Source: CAD feature listing. Evaluate the final solid. Frame: model axes, mm. A direction names the side the tool comes from. Coordinates: 2 decimals unless noted, no trailing zeros. Write each loop counter-clockwise with the first axis right and the second up, starting at its lowest first coordinate (ties: lowest second). Pieces come first, ordered by that corner, then holes. Notation, with made-up numbers: (-13, 11) - (16, 11) arc R13 cw to (16, 20) - close; hole circle Ø8 at (28.5, -38). An arc over 180 degrees is marked (long way). One line per question, with ' | ' between items. Start each with the question number.
Q1. Cut plane B-B, the plane x = -178.5. Return loops of the section in (y, z), plus the area to 3 significant figures.
Q2. Access query for faces 1 (the face through (-4, 1.143, -1)), 2 (the face through (4, -1.143, -1)). Directions: +Z, -Z, +X, -X, +Y, -Y. A direction counts if a zero-diameter tool reaches every point of the face in a straight line with its end or side. Return the directions, or none.
Q3. Cut plane D-D, the plane x = 21. Return loops of the section in (y, z), plus the area to 3 significant figures.
Q4. Cut plane A-A, the plane z = -6.5. Return loops of the section in (x, y).
Q5. Cut plane C-C, the plane z = 51.5. Return loops of the section in (x, y).
Q6. Line query: line 1 (X direction, y = -0.85, z = -31); line 2 (Y direction, x = 54.5, z = -42); line 3 (X direction, y = 0.2, z = 36). Output: solid intervals per line, ascending.
Q7. Contact query for flat-ended pins moving along their axis: P1, Ø0.8, axis at y = 0, z = -75, coming from the +X side; P2, Ø1.1, axis at x = -317, y = 0.5, coming from the +Z side; P3, Ø0.7, axis at x = 18.5, y = 0, coming from the -Z side. Output: stop coordinate, or through.
```python
from build123d import *

# Parameters (mm, degrees)
SKETCH1_W           = 635.3556
SKETCH1_H           = 145.542
BOSS_EXTRUDE1_DEPTH = 1.143
SKETCH2_W           = 254
SKETCH2_H           = 2.7305
BOSS_EXTRUDE2_DEPTH = 3.175
SKETCH3_W           = 3.175
SKETCH3_H           = 38.1
CUT_EXTRUDE1_DEPTH  = 3.7305
SKETCH4_W           = 2.3368
SKETCH4_H           = 72.771
CUT_EXTRUDE2_DEPTH  = 3.7305


with BuildPart() as part:
    # Sketch1 → Boss-Extrude1 (new body, symmetric)
    with BuildSketch(Plane(origin=(0, 0, 0), x_dir=(1, 0, 0), z_dir=(0, 1, 0))):
        Rectangle(SKETCH1_W, SKETCH1_H)
    extrude(amount=BOSS_EXTRUDE1_DEPTH, both=True)

    # Sketch2 → Boss-Extrude2 (add)
    with BuildSketch(Plane(origin=(0, 0, -72.771), x_dir=(-1, 0, 0), z_dir=(0, 0, -1))):
        with Locations((-157.8229, 0.22225)):
            Rectangle(SKETCH2_W, SKETCH2_H)
        with Locations((157.8229, 0.22225)):
            Rectangle(SKETCH2_W, SKETCH2_H)
    extrude(amount=BOSS_EXTRUDE2_DEPTH)

    # Sketch3 → Cut-Extrude1 (cut, through all)
    with BuildSketch(Plane.XZ.offset(1.143)):
        with Locations((-316.0903, 53.721)):
            Rectangle(SKETCH3_W, SKETCH3_H)
    cut_extrude1 = extrude(amount=-CUT_EXTRUDE1_DEPTH, mode=Mode.SUBTRACT)

    # Mirror1: Cut-Extrude1 across plane
    add(cut_extrude1.mirror(Plane(origin=(0, 0, 0), x_dir=(0, 0, 1), z_dir=(1, 0, 0))), mode=Mode.SUBTRACT)

    # Sketch4 → Cut-Extrude2 (cut, through all)
    with BuildSketch(Plane.XZ.offset(1.143)):
        with Locations((0.0254, -36.3855)):
            Rectangle(SKETCH4_W, SKETCH4_H)
    extrude(amount=-CUT_EXTRUDE2_DEPTH, mode=Mode.SUBTRACT)


solid = part.part
```
Reply:
1) outline: (-1.14, -75.95) - (1.59, -75.95) - (1.59, -72.77) - (1.14, -72.77) - (1.14, 72.77) - (-1.14, 72.77) - close | area: 341 mm^2
2) face 1: +Z, +X, -X, +Y | face 2: +Z, -Z, +X, -X, -Y
3) outline: (-1.14, -72.77) - (1.14, -72.77) - (1.14, 72.77) - (-1.14, 72.77) - close | area: 333 mm^2
4) outline: (-317.68, -1.14) - (-1.14, -1.14) - (-1.14, 1.14) - (-317.68, 1.14) - close; (1.19, -1.14) - (317.68, -1.14) - (317.68, 1.14) - (1.19, 1.14) - close
5) outline: (-314.5, -1.14) - (314.5, -1.14) - (314.5, 1.14) - (-314.5, 1.14) - close
6) line 1: x = -317.68 to -1.14, 1.19 to 317.68 | line 2: y = -1.14 to 1.14 | line 3: x = -314.5 to 314.5
7) P1: stops at x = 284.82 | P2: stops at z = 34.67 | P3: stops at z = -72.77
